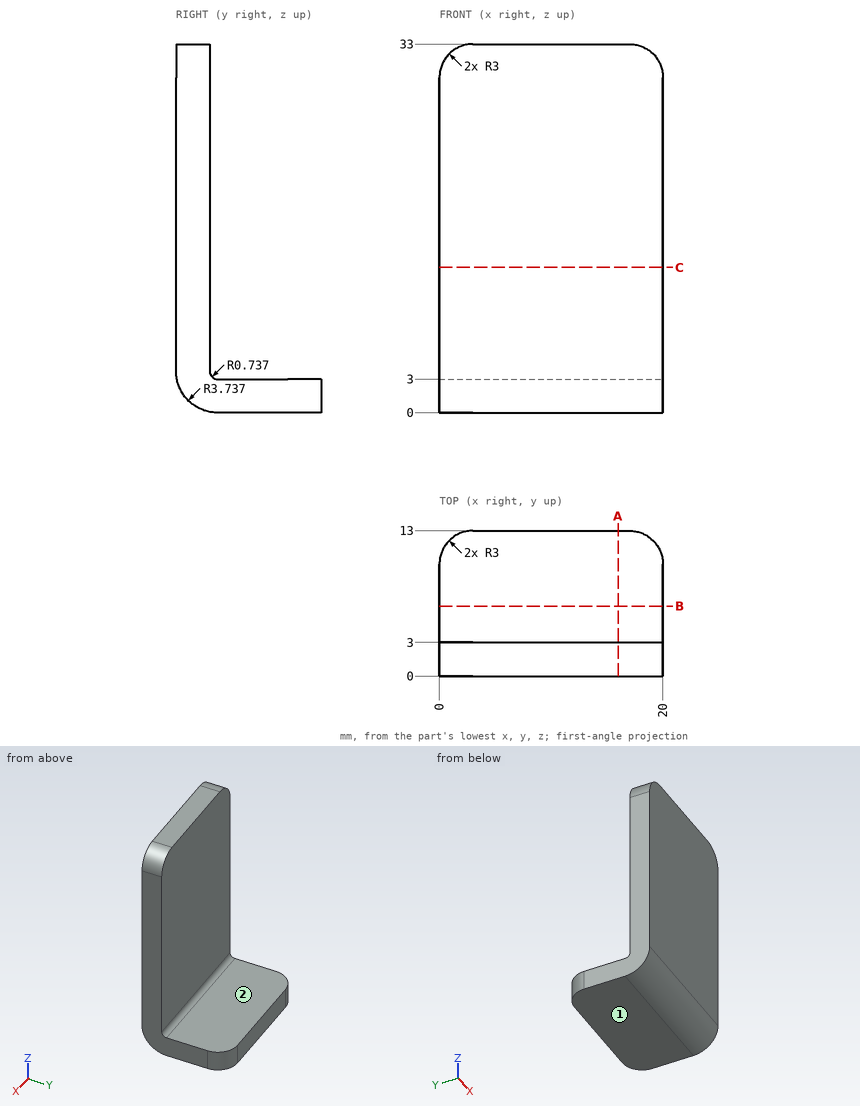
Design review of the part shown in the three views and the two pictorial views. Dimensions are in mm from the part's minimum x, y and z. A direction names the side the tool comes from. Coordinates: 2 decimals unless noted, no trailing zeros. Loops run counter-clockwise (first coordinate to the right, second up) from the corner with the lowest first, then second, coordinate; pieces in that order, holes last.
(1) Insertion check: P1, Ø6, axis at x = 8.5, z = 24, coming from the +Y side; P2, Ø7.5, axis at x = 12.5, y = 10.5, coming from the +Z side. Each pin has a flat end and moves straight along its axis. Give the tip position at first contact, or say it passes through.
Determined:
P1: stops at y = 3
P2: stops at z = 3
(2) Consider section B-B, the plane y = 6.25. Give the boundary of the cut face in (x, z), plus the area to 3 significant figures.
Determined:
outline: (0, 0) - (20, 0) - (20, 3) - (0, 3) - close
area: 60.0 mm2
(3) Tool access review of the marked faces 1 and 2: name each direction out of +Z, -Z, +X, -X, +Y, -Y from which nothing blocks a thin tool from reaching the whole face with its end or side.
Determined:
face 1: -Z, +X, -X, +Y, -Y
face 2: +Z, +X, -X, +Y
(4) Consider section A-A, the plane x = 16. Give the boundary of the cut face in (y, z).
Determined:
outline: (0, 3.74) arc R3.74 ccw to (3.74, 0) - (13, 0) - (13, 3) - (3.74, 3) arc R0.74 cw to (3, 3.74) - (3, 33) - (0, 33) - close
(5) Wall thickness on L1, parallel to Y at x = 9, z = 4.5; L2, parallel to Z at x = 11.5, y = 2.25: over which ranges is each line inside the solid? List them lowest first.
Determined:
L1: y = 0 to 3
L2: z = 0.31 to 33
